Model file for the job. Use its own axes, mm. Face numbers are marked on the shaded views. A direction names the side the tool comes from. Round coordinates to 2 decimals unless told otherwise and drop trailing zeros. Loops run counter-clockwise (first coordinate to the right, second up) from the corner with the lowest first, then second, coordinate; pieces in that order, holes last. Notation, with made-up numbers: (32.25, -24.5) - (72.25, -24.5) arc R26 ccw to (72.25, 9.5) - close; hole circle Ø8 at (42.5, -19). An arc over 180 degrees is marked (long way). Answer as a JSON object with one key per item and string values.
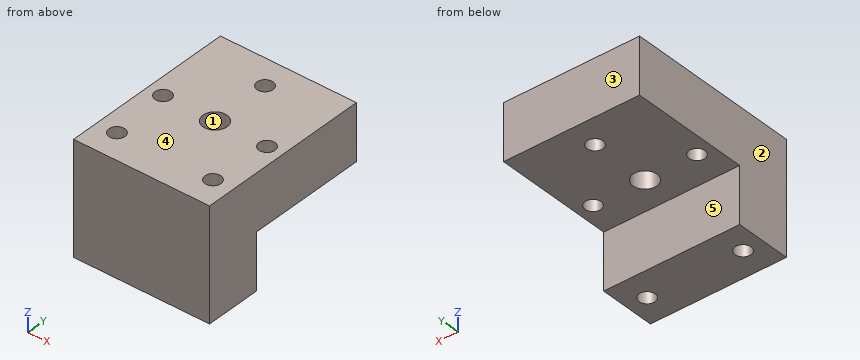
from build123d import *

# Parameters (mm, degrees)
SKETCH1_W           = 215.9
SKETCH1_H           = 101.6
SKETCH1_R           = 12.7
SKETCH1_H_2         = 88.9
BOSS_EXTRUDE1_DEPTH = 88.9
SKETCH1_3_W         = 215.9
SKETCH1_3_H         = 88.9
BOSS_EXTRUDE2_DEPTH = 88.9
SKETCH2_W           = 215.9
SKETCH2_H           = 88.9
SKETCH2_R           = 12.7
BOSS_EXTRUDE3_DEPTH = 88.9
CUT_EXTRUDE1_REACH  = 252.564
SKETCH2_3_R         = 12.7
SKETCH2_3_R_2       = 19.05


with BuildPart() as part:
    # Sketch1 → Boss-Extrude1 (new body)
    # profile 1 of 2: a face of its own
    with BuildSketch(Plane.XY):
        Rectangle(SKETCH1_W, SKETCH1_H)
        with Locations((82.55, 0)):
            Circle(SKETCH1_R, mode=Mode.SUBTRACT)
        with Locations((-82.55, 0)):
            Circle(SKETCH1_R, mode=Mode.SUBTRACT)
    # profile 2 of 2: a face of its own
    with BuildSketch(Plane.XY):
        with Locations((0, -95.25)):
            Rectangle(SKETCH1_W, SKETCH1_H_2)
    extrude(amount=BOSS_EXTRUDE1_DEPTH)

    # Sketch1<3> → Boss-Extrude2 (add)
    with BuildSketch(Plane.XY):
        with Locations((0, -95.25)):
            Rectangle(SKETCH1_3_W, SKETCH1_3_H)
    extrude(amount=-BOSS_EXTRUDE2_DEPTH)

    # Sketch2 → Boss-Extrude3 (add)
    with BuildSketch(Plane.XY.offset(88.9)):
        with Locations((0, 95.25)):
            Rectangle(SKETCH2_W, SKETCH2_H)
        with Locations((0, 95.25)):
            Circle(SKETCH2_R, mode=Mode.SUBTRACT)
    extrude(amount=-BOSS_EXTRUDE3_DEPTH)

    # Sketch2<3> → Cut-Extrude1 (cut, up to next)
    with BuildSketch(Plane.XY.offset(88.9), mode=Mode.PRIVATE) as cut_extrude1_sk1:
        with Locations((-76.2, -95.25)):
            Circle(SKETCH2_3_R)
    cut_extrude1_tool1 = extrude(cut_extrude1_sk1.sketch, amount=-CUT_EXTRUDE1_REACH, mode=Mode.PRIVATE) & part.part
    # Sketch2<3> → Cut-Extrude1 (cut, up to next)
    with BuildSketch(Plane.XY.offset(88.9), mode=Mode.PRIVATE) as cut_extrude1_sk2:
        with Locations((76.2, -95.25)):
            Circle(SKETCH2_3_R)
    cut_extrude1_tool2 = extrude(cut_extrude1_sk2.sketch, amount=-CUT_EXTRUDE1_REACH, mode=Mode.PRIVATE) & part.part
    # Sketch2<3> → Cut-Extrude1 (cut, up to next)
    with BuildSketch(Plane.XY.offset(88.9), mode=Mode.PRIVATE) as cut_extrude1_sk3:
        Circle(SKETCH2_3_R_2)
    cut_extrude1_tool3 = extrude(cut_extrude1_sk3.sketch, amount=-CUT_EXTRUDE1_REACH, mode=Mode.PRIVATE) & part.part
    add(cut_extrude1_tool1.solids().sort_by_distance((-76.2, -95.25, 88.9))[0], mode=Mode.SUBTRACT)
    add(cut_extrude1_tool2.solids().sort_by_distance((76.2, -95.25, 88.9))[0], mode=Mode.SUBTRACT)
    add(cut_extrude1_tool3.solids().sort_by_distance((0, 0, 88.9))[0], mode=Mode.SUBTRACT)


solid = part.part
1) Probe probe 1 along X at (y, z) = (-95, -29); probe 2 along Y at (x, z) = (0, 60); probe 3 along Y at (x, z) = (78, 44.5). List the from-to ranges inside material, lowest first.
Values follow:
{"probe 1": "-107.95 to -88.9, -63.5 to 63.5, 88.9 to 107.95", "probe 2": "-139.7 to -19.05, 19.05 to 82.55, 107.95 to 139.7", "probe 3": "-139.7 to -107.82, -82.68 to -11.86, 11.86 to 139.7"}
2) Slice it at D-D on x = -39. List the corners of the cut face in (y, z).
Values follow:
{"outline": "(-139.7, -88.9) - (-50.8, -88.9) - (-50.8, 0) - (139.7, 0) - (139.7, 88.9) - (-139.7, 88.9) - close"}
3) Drop flat-ended pins along their axis: P1, Ø5, axis at x = -69, y = -104, coming from the +Z side; P2, Ø15, axis at x = 0, y = 95.25, coming from the -Z side; P3, Ø5, axis at x = 68.5, y = 5.5, coming from the -Z side. Give the stop position or say it passes through.
Values follow:
{"P1": "z = 88.9", "P2": "through", "P3": "z = 0"}
4) Tool access for the marked faces 4 and 5: list every direction of +Z, -Z, +X, -X, +Y, -Y with a clear straight run to the whole face (end or side of a thin tool).
Values follow:
{"face 4": "+Z, +X, -X, +Y, -Y", "face 5": "-Z, +X, -X, +Y"}
5) Two-plate mould, pull along X, no slides. Class the marked faces 1, 2 and 3: pulls with the +X half, pulls with the -X half, needs draft (parallel to the pull), parting line crosses it, or undercut.
Values follow:
{"face 1": "undercut", "face 2": "pulls with the -X half", "face 3": "needs draft"}
6) Slice it at B-B on z = 57. List the corners of the cut face in (x, y), then the cut area to 3 significant figures.
Values follow:
{"outline": "(-107.95, -139.7) - (107.95, -139.7) - (107.95, 139.7) - (-107.95, 139.7) - close; hole circle Ø25.4 at (-82.55, 0); hole circle Ø25.4 at (-76.2, -95.25); hole circle Ø38.1 at (0, 0); hole circle Ø25.4 at (0, 95.25); hole circle Ø25.4 at (76.2, -95.25); hole circle Ø25.4 at (82.55, 0)", "area": "56,600 mm²"}
7) Slice it at C-C on y = 95.25. List the corners of the cut face in (x, z).
Values follow:
{"outline": "(-107.95, 0) - (-12.7, 0) - (-12.7, 88.9) - (-107.95, 88.9) - close; (12.7, 0) - (107.95, 0) - (107.95, 88.9) - (12.7, 88.9) - close"}
8) Slice it at A-A on x = 0. List the corners of the cut face in (y, z).
Values follow:
{"outline": "(-139.7, -88.9) - (-50.8, -88.9) - (-50.8, 0) - (-19.05, 0) - (-19.05, 88.9) - (-139.7, 88.9) - close; (19.05, 0) - (82.55, 0) - (82.55, 88.9) - (19.05, 88.9) - close; (107.95, 0) - (139.7, 0) - (139.7, 88.9) - (107.95, 88.9) - close"}
